Design review of the part built by this model. Coordinates are the model's own, in mm. A direction names the side the tool comes from. Give positions to 0.01 mm unless a question says otherwise; leave off trailing zeros. Loops run counter-clockwise (first coordinate to the right, second up) from the corner with the lowest first, then second, coordinate; pieces in that order, holes last. Notation, with made-up numbers: (-25, 75) - (15, 75) arc R24 ccw to (15, 110) - close; hole circle Ø9 at (-12, 0). An arc over 180 degrees is marked (long way). One line per item, written item: value. Start each with the question number.
```python
from build123d import *

# Parameters (mm, degrees)
F0_W     = 32.16
F0_H     = 31
F1_DEPTH = 12.5
F2_T     = -3
F3_W     = 17.16
F3_H     = 3
F4_DEPTH = 10
F6_D     = 8
F6_DEPTH = 5
F6_TIP   = 2.4034424761
F8_D     = 2.1
F8_DEPTH = 5
F8_TIP   = 0.63090365


with BuildPart() as f1:
    # F0 (on Top) → F1 (new body)
    with BuildSketch(Plane.XY):
        Rectangle(F0_W, F0_H)
    extrude(amount=F1_DEPTH)

    # F2
    f2_openings = [f1.faces().sort_by_distance(p)[0] for p in [
        (0, 0, 12.5),
    ]]
    offset(amount=F2_T, openings=f2_openings)

    # F3 (on face) → F4 (cut)
    with BuildSketch(Plane.XY.offset(12.5)):
        with Locations((0, -14)):
            Rectangle(F3_W, F3_H)
    extrude(amount=-F4_DEPTH, mode=Mode.SUBTRACT)

    # F6
    with Locations(Plane.XY.offset(3)):
        with Locations((0, 4.65)):
            Hole(F6_D / 2, depth=F6_DEPTH)
            with Locations((0, 0, -(F6_DEPTH + F6_TIP / 2))):  # 118° drill point
                Cone(0, F6_D / 2, F6_TIP, mode=Mode.SUBTRACT)

    # F8
    with Locations(Plane.XY.offset(12.5)):
        with Locations((-14.2255129855, -13.6455129855), (14.2255129855, -13.6455129855), (14.2255129855, 13.6455129855), (-14.2255129855, 13.6455129855)):
            Hole(F8_D / 2, depth=F8_DEPTH)
            with Locations((0, 0, -(F8_DEPTH + F8_TIP / 2))):  # 118° drill point
                Cone(0, F8_D / 2, F8_TIP, mode=Mode.SUBTRACT)


solid = f1.part
```
(1) Draft analysis for pull direction Y (two halves, no side actions). For faces 1 (the flat face through (-16.08, 0, 6)), 2 (the flat face through (0, 15.5, 6)), 3 (the flat face through (-11, -12.5, 8)), state which applies: pulls with the +Y half, pulls with the -Y half, needs draft (parallel to the pull), parting line crosses it, or undercut.
(2) Take a section at C-C on x = -4.5. State the section outline as (y, z) points, and give its area (3 significant figures).
(3) For pin 1 Ø5 at (x, y) = (0.5, -10.5) entering from -Z; pin 2 Ø1.7 at (x, y) = (-14.23, -13.65) entering from +Z; pin 3 Ø5 at (x, y) = (-4.5, 2) entering from +Z; pin 4 Ø0.9 at (x, y) = (-3.5, -13.5) entering from +Z, all flat-tipped, find the tip position at first contact; note any pin that passes through.
(4) Take a section at D-D on z = 9. State the section outline as (x, y) points.
(5) Machinability: for faces 4 (the cylindrical face through (-15.227, 13.961, 9.965)), 5 (the flat face through (8.58, -14, 8)), 6 (the flat face through (16.08, 0, 6)), which of the approach directions +Z, -Z, +X, -X, +Y, -Y give a long, thin tool a straight path to every point of the face, cutting with its end or side? Answer none if there is none.
(6) Take a section at B-B on x = 0. State the section outline as (y, z) points.
(7) To check wall thickness, follow L1, parallel to X at y = -14, z = 9.25; L2, parallel to X at y = -12, z = 7.5; L3, parallel to Y at x = -9.5, z = 7.25. State the ranges of each line that lie inside material, in increasing order. Write a range as from..to.
(8) Take a section at A-A on y = 4.65. State the section outline as (x, z) points.
Here are the results:
1. face 1: needs draft
1. face 2: pulls with the +Y half
1. face 3: undercut
2. outline: (-15.5, 0) - (15.5, 0) - (15.5, 12.5) - (12.5, 12.5) - (12.5, 3) - (-12.5, 3) - (-12.5, 2.5) - (-15.5, 2.5) - close
2. area: 120 mm²
3. pin 1: z = 0
3. pin 2: z = 7.38
3. pin 3: z = 3
3. pin 4: z = 2.5
4. outline: (-16.08, -15.5) - (-8.58, -15.5) - (-8.58, -12.5) - (-13.08, -12.5) - (-13.08, 12.5) - (13.08, 12.5) - (13.08, -12.5) - (8.58, -12.5) - (8.58, -15.5) - (16.08, -15.5) - (16.08, 15.5) - (-16.08, 15.5) - close; hole circle Ø2.1 at (-14.23, -13.65); hole circle Ø2.1 at (-14.23, 13.65); hole circle Ø2.1 at (14.23, -13.65); hole circle Ø2.1 at (14.23, 13.65)
5. face 4: +Z
5. face 5: +Z, -Y
5. face 6: +Z, -Z, +X, +Y, -Y
6. outline: (-15.5, 0) - (0.65, 0) - (0.65, 3) - (-12.5, 3) - (-12.5, 2.5) - (-15.5, 2.5) - close; (8.65, 0) - (15.5, 0) - (15.5, 12.5) - (12.5, 12.5) - (12.5, 3) - (8.65, 3) - close
7. L1: -16.08..-15.21, -13.24..-8.58, 8.58..13.24, 15.21..16.08
7. L2: -16.08..-13.08, 13.08..16.08
7. L3: -15.5..-12.5, 12.5..15.5
8. outline: (-16.08, 0) - (-4, 0) - (-4, 3) - (-13.08, 3) - (-13.08, 12.5) - (-16.08, 12.5) - close; (4, 0) - (16.08, 0) - (16.08, 12.5) - (13.08, 12.5) - (13.08, 3) - (4, 3) - close
